Input: part model. Units: mm. Frame: model coordinates. Face numbers are marked on the shaded views. A direction names the side the tool comes from. Coordinates: 2 decimals unless noted, no trailing zeros. Order: outer loops, then holes, each group sorted by start corner. A loop starts at its lowest first (then second) coordinate and runs counter-clockwise, first axis right, second up. Notation, with made-up numbers: (56, 14) -> (110, 14) arc R17 ccw to (110, 47) -> close; hole circle Ø3 at (88, 5.5). An arc over 180 degrees is marked (long way). Answer as CSV lines item,"result".
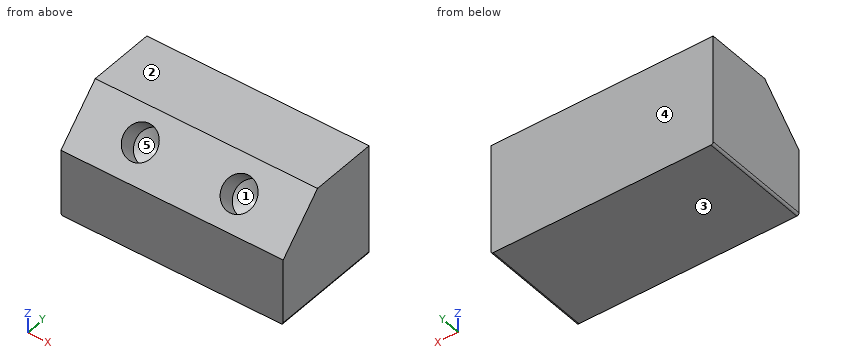
from build123d import *

# Parameters (mm, degrees)
F0_W     = 100
F0_H     = 50
F1_DEPTH = 50
F2_SIZE  = 20
F5_D     = 15
F5_DEPTH = 10
F5_TIP   = 4.5064546427
F6_D     = 15
F6_DEPTH = 10
F6_TIP   = 4.5064546427
F7_R     = 1


with BuildPart() as f1:
    # F0 (on Top) → F1 (new body)
    with BuildSketch(Plane.XY):
        with Locations((-50, -25)):
            Rectangle(F0_W, F0_H)
    extrude(amount=F1_DEPTH)

    # F2
    f2_edges = [f1.edges().sort_by_distance(p)[0] for p in [
        (-50, -50, 50),
    ]]
    chamfer(f2_edges, length=F2_SIZE)

    # F5
    with Locations(Plane(origin=(0, -40, 40), x_dir=(1, 0, 0), z_dir=(0, -0.7071067812, 0.7071067812))):
        with Locations((-27.5615938008, 0)):
            Hole(F5_D / 2, depth=F5_DEPTH)
            with Locations((0, 0, -(F5_DEPTH + F5_TIP / 2))):  # 118° drill point
                Cone(0, F5_D / 2, F5_TIP, mode=Mode.SUBTRACT)

    # F6
    with Locations(Plane(origin=(0, -40, 40), x_dir=(1, 0, 0), z_dir=(0, -0.7071067812, 0.7071067812))):
        with Locations((-72.5, 0.8578643763)):
            Hole(F6_D / 2, depth=F6_DEPTH)
            with Locations((0, 0, -(F6_DEPTH + F6_TIP / 2))):  # 118° drill point
                Cone(0, F6_D / 2, F6_TIP, mode=Mode.SUBTRACT)

    # F7
    f7_edges = [f1.edges().sort_by_distance(p)[0] for p in [
        (0, -25, 0),
        (-100, -25, 0),
    ]]
    fillet(f7_edges, radius=F7_R)


solid = f1.part
1. Reachability of the marked faces 1 and 2 from +Z, -Z, +X, -X, +Y, -Y: full face, straight path, thin tool, end or side. Return the list, or none.
Findings:
face 1,"none"
face 2,"+Z, +X, -X, +Y, -Y"
2. Mould query, pull axis Z, two halves, no side actions, for the marked faces 3, 4 and 5. Classes: released by +Z, released by -Z, zero draft, split by the parting line, or undercut.
Findings:
face 3,"released by -Z"
face 4,"zero draft"
face 5,"undercut"
3. Ray query, line 1 along Z through (x, y) = (-28, -36); line 2 along Z through (x, y) = (-30.5, -48); line 3 along Y through (x, z) = (-14.5, 43). Return the intervals inside material, ascending.
Findings:
line 1,"z = 0 to 28.19"
line 2,"z = 0 to 32"
line 3,"y = -37 to 0"
4. Contact query for a flat-ended pin moving along its axis: pin 1 (5 mm diameter, centred on x = -42, y = -36.5, fed in from +Z). Output: stop coordinate, or through.
Findings:
pin 1,"stops at z = 46"
5. Cut plane A-A (x = -44.5). Return the cut outline in (y, z).
Findings:
outline,"(-50, 0) -> (0, 0) -> (0, 50) -> (-30, 50) -> (-50, 30) -> close"
